Design review of the part built by this model. Coordinates are the model's own, in mm. Face numbers are marked on the shaded views. A direction names the side the tool comes from. Give positions to 0.01 mm unless a question says otherwise; leave off trailing zeros. Loops run counter-clockwise (first coordinate to the right, second up) from the corner with the lowest first, then second, coordinate; pieces in that order, holes last. Notation, with made-up numbers: (44, -29) - (74, -29) arc R32 cw to (74, 9) - close; hole circle Ø9 at (40, 36). An arc over 180 degrees is marked (long way). Write each question's results on one line, items separated by ' | '.
```python
from build123d import *

# Parameters (mm, degrees)
SKETCH_W        = 85
SKETCH_H        = 110
PAD_DEPTH       = 3.5
SKETCH001_W     = 85
SKETCH001_H     = 110
PAD001_DEPTH    = 17.5
SKETCH002_W     = 81
SKETCH002_H     = 106
POCKET_DEPTH    = 17.5
SKETCH003_W     = 85
SKETCH003_H     = 110
SKETCH003_W_2   = 83
SKETCH003_H_2   = 108
POCKET001_DEPTH = 2.5
SKETCH004_R     = 9
SKETCH004_W     = 14
SKETCH004_H     = 12
POCKET002_DEPTH = 5
SKETCH005_R     = 8
SKETCH005_W     = 13
SKETCH005_H     = 12
POCKET003_DEPTH = 5
SKETCH006_R     = 2.25
POCKET004_DEPTH = 5
SKETCH007_R     = 6.5
POCKET005_DEPTH = 5


with BuildPart() as part:
    # Sketch → Pad (new body)
    with BuildSketch(Plane.XY):
        Rectangle(SKETCH_W, SKETCH_H)
    extrude(amount=PAD_DEPTH)

    # Sketch001 (on Face6 of Pad) → Pad001 (join)
    with BuildSketch(Plane.XY.offset(3.5)):
        Rectangle(SKETCH001_W, SKETCH001_H)
    extrude(amount=PAD001_DEPTH)

    # Sketch002 (on Face9 of Pad001) → Pocket (cut)
    with BuildSketch(Plane.XY.offset(21)):
        Rectangle(SKETCH002_W, SKETCH002_H)
    extrude(amount=-POCKET_DEPTH, mode=Mode.SUBTRACT)

    # Sketch003 (on Face9 of Pocket) → Pocket001 (cut)
    with BuildSketch(Plane.XY.offset(21)):
        Rectangle(SKETCH003_W, SKETCH003_H)
        Rectangle(SKETCH003_W_2, SKETCH003_H_2, mode=Mode.SUBTRACT)
    extrude(amount=-POCKET001_DEPTH, mode=Mode.SUBTRACT)

    # Sketch004 (on Face10 of Pocket001) → Pocket002 (cut)
    with BuildSketch(Plane.XZ.offset(55)):
        with Locations((12.67, 20.5)):
            Circle(SKETCH004_R)
        with Locations((-18.67, 23.5)):
            Rectangle(SKETCH004_W, SKETCH004_H)
    extrude(amount=-POCKET002_DEPTH, mode=Mode.SUBTRACT)

    # Sketch005 (on Face5 of Pocket002) → Pocket003 (cut)
    with BuildSketch(Plane(origin=(0, 55, 0), x_dir=(-1, 0, 0), z_dir=(0, 1, 0))):
        with Locations((-1.33, 18.5)):
            Circle(SKETCH005_R)
        with Locations((16.17, 23.5)):
            Rectangle(SKETCH005_W, SKETCH005_H)
    extrude(amount=-POCKET003_DEPTH, mode=Mode.SUBTRACT)

    # Sketch006 (on Face39 of Pocket003) → Pocket004 (cut)
    with BuildSketch(Plane.XY.offset(3.5)):
        with Locations((-36.21, 48.71)):
            Circle(SKETCH006_R)
        with Locations((36.21, 48.71)):
            Circle(SKETCH006_R)
        with Locations((-36.21, -48.71)):
            Circle(SKETCH006_R)
        with Locations((36.21, -48.71)):
            Circle(SKETCH006_R)
    extrude(amount=-POCKET004_DEPTH, mode=Mode.SUBTRACT)

    # Sketch007 (on Face21 of Pocket004) → Pocket005 (cut)
    with BuildSketch(Plane.XY.offset(3.5)):
        Circle(SKETCH007_R)
    extrude(amount=-POCKET005_DEPTH, mode=Mode.SUBTRACT)


solid = part.part
```
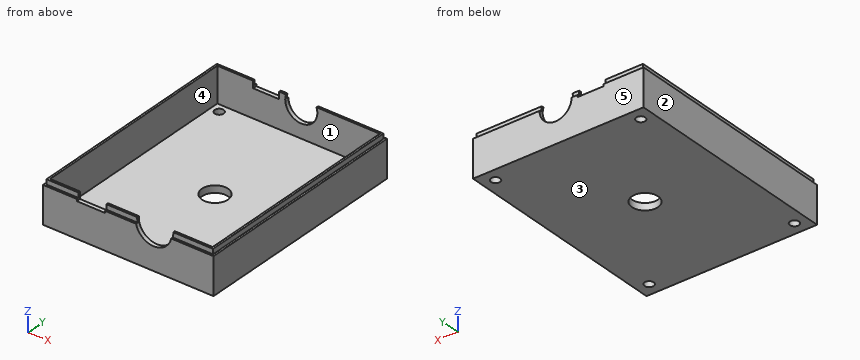
Item 1: Clearance check with flat-ended pins moving along their axes: P1, Ø17, axis at x = 0, y = 0, coming from the -Z side; P2, Ø0.8, axis at x = -7.5, y = 54.5, coming from the +Z side; P3, Ø1.2, axis at x = -31, z = 20.5, coming from the -Y side; P4, Ø9.5, axis at x = 1.33, z = 18.5, coming from the +Y side. State where each tip first meets the part, or that it passes through.
Output values:
P1: stops at z = 0 | P2: stops at z = 18.5 | P3: stops at y = -54 | P4: stops at y = -53
Item 2: We need section D-D on y = 0. Give the boundary of the cut face in (x, z).
Output values:
outline: (-42.5, 0) - (-6.5, 0) - (-6.5, 3.5) - (-40.5, 3.5) - (-40.5, 21) - (-41.5, 21) - (-41.5, 18.5) - (-42.5, 18.5) - close; (6.5, 0) - (42.5, 0) - (42.5, 18.5) - (41.5, 18.5) - (41.5, 21) - (40.5, 21) - (40.5, 3.5) - (6.5, 3.5) - close
Item 3: Draft analysis for pull direction Y (two halves, no side actions). For the marked faces 3, 4 and 5, state which applies: +Y half, -Y half, draft (parallel to the pull), parting line (faces both ways), or undercut.
Output values:
face 3: draft | face 4: undercut | face 5: +Y half
Item 4: We need section C-C on z = 13.25. Give the boundary of the cut face in (x, y), then the cut area to 3 significant figures.
Output values:
outline: (-42.5, -55) - (7.34, -55) - (7.34, -53) - (-40.5, -53) - (-40.5, 53) - (-4.71, 53) - (-4.71, 55) - (-42.5, 55) - close; (7.37, 53) - (40.5, 53) - (40.5, -53) - (18, -53) - (18, -55) - (42.5, -55) - (42.5, 55) - (7.37, 55) - close | area: 719 mm²
Item 5: Wall thickness on probe 1 along Y at (x, z) = (-36.21, 2.3); probe 2 along Y at (x, z) = (0, 2.7); probe 3 along X at (y, z) = (5, 5): over which ranges is each line inside the solid? List them lowest first.
Output values:
probe 1: y = -55 to -50.96, -46.46 to 46.46, 50.96 to 55 | probe 2: y = -55 to -6.5, 6.5 to 55 | probe 3: x = -42.5 to -40.5, 40.5 to 42.5
Item 6: We need section A-A on x = 36.21. Give the boundary of the cut face in (y, z).
Output values:
outline: (-55, 0) - (-50.96, 0) - (-50.96, 3.5) - (-53, 3.5) - (-53, 21) - (-54, 21) - (-54, 18.5) - (-55, 18.5) - close; (-46.46, 0) - (46.46, 0) - (46.46, 3.5) - (-46.46, 3.5) - close; (50.96, 0) - (55, 0) - (55, 18.5) - (54, 18.5) - (54, 21) - (53, 21) - (53, 3.5) - (50.96, 3.5) - close
Item 7: Tool access review of the marked faces 1 and 2: name each direction out of +Z, -Z, +X, -X, +Y, -Y from which nothing blocks a thin tool from reaching the whole face with its end or side.
Output values:
face 1: +Z | face 2: +Z, -Z, -X, +Y, -Y
Item 8: We need section B-B on y = 48.71. Give the boundary of the cut face in (x, z).
Output values:
outline: (-42.5, 0) - (-38.46, 0) - (-38.46, 3.5) - (-40.5, 3.5) - (-40.5, 21) - (-41.5, 21) - (-41.5, 18.5) - (-42.5, 18.5) - close; (-33.96, 0) - (33.96, 0) - (33.96, 3.5) - (-33.96, 3.5) - close; (38.46, 0) - (42.5, 0) - (42.5, 18.5) - (41.5, 18.5) - (41.5, 21) - (40.5, 21) - (40.5, 3.5) - (38.46, 3.5) - close
